from build123d import *

# Parameters (mm, degrees)
SKETCH1_R                = 0.15
BOSS_EXTRUDE1_DEPTH      = 0.1
SKETCH2_R                = 0.3
SKETCH2_R_2              = 0.15
BOSS_EXTRUDE2_DEPTH      = 0.1
BOSS_EXTRUDE2_DEPTH_BACK = 2
FILLET1_R                = 0.05
FILLET2_R                = 0.02
SKETCH3_R                = 0.431407551
SKETCH3_R_2              = 0.2
CUT_EXTRUDE1_DEPTH       = 1.9


with BuildPart() as part:
    # Sketch1 → Boss-Extrude1 (new body)
    with BuildSketch(Plane(origin=(0, 0, 0), x_dir=(1, 0, 0), z_dir=(0, 1, 0))):
        with BuildLine():
            Line((-82.406253285, -49.725868429), (-72.592962822, -38.875374501))
            ThreePointArc((-72.592962822, -38.875374501), (-71.888648973, -38.644732606), (-71.760288486, -37.914816674))
            Line((-71.760288486, -37.914816674), (-69.191054527, -35.004040233))
            Line((-69.191054527, -35.004040233), (-69.671325788, -34.569459042))
            Line((-69.671325788, -34.569459042), (-72.275341711, -37.469639173))
            ThreePointArc((-72.275341711, -37.469639173), (-72.996004438, -37.722822834), (-73.084190733, -38.481558565))
            Line((-73.084190733, -38.481558565), (-82.643859616, -49.510974991))
            Line((-82.643859616, -49.510974991), (-82.406253285, -49.725868429))
        make_face()
        with Locations((-72.433134731, -38.172736745)):
            Circle(SKETCH1_R, mode=Mode.SUBTRACT)
    extrude(amount=BOSS_EXTRUDE1_DEPTH)

    # Sketch2 → Boss-Extrude2 (add, two sides)
    with BuildSketch(Plane(origin=(0, 0.1, 0), x_dir=(1, 0, 0), z_dir=(0, 1, 0))) as boss_extrude2_sk:
        with Locations((-72.433134731, -38.172736745)):
            Circle(SKETCH2_R)
        with Locations((-72.433134731, -38.172736745)):
            Circle(SKETCH2_R_2, mode=Mode.SUBTRACT)
    extrude(amount=BOSS_EXTRUDE2_DEPTH)
    extrude(boss_extrude2_sk.sketch, amount=-BOSS_EXTRUDE2_DEPTH_BACK)

    # Fillet1
    fillet1_edges = [part.edges().sort_by_distance(p)[0] for p in [
        (-72.583134731, 0.2, 38.172736745),
        (-72.733134731, 0.2, 38.172736745),
    ]]
    fillet(fillet1_edges, radius=FILLET1_R)

    # Fillet2
    fillet2_edges = [part.edges().sort_by_distance(p)[0] for p in [
        (-77.499608053, 0.1, 44.300621465),
        (-71.888648973, 0.1, 38.644732606),
        (-70.475671506, 0.1, 36.459428453),
        (-69.431190157, 0.1, 34.786749638),
        (-70.973333749, 0.1, 36.019549108),
        (-72.733134731, 0.1, 38.172736745),
        (-72.996004438, 0.1, 37.722822834),
        (-77.864025175, 0.1, 43.996266778),
        (-82.52505645, 0.1, 49.61842171),
    ]]
    fillet(fillet2_edges, radius=FILLET2_R)

    # Sketch3 → Cut-Extrude1 (cut)
    with BuildSketch(Plane.XZ.offset(1.9)):
        with Locations((-72.433134731, 38.172736745)):
            Circle(SKETCH3_R)
        with Locations((-72.433134731, 38.172736745)):
            Circle(SKETCH3_R_2, mode=Mode.SUBTRACT)
    extrude(amount=-CUT_EXTRUDE1_DEPTH, mode=Mode.SUBTRACT)


solid = part.part
The listing builds one solid part. Answer for the finished solid, in the listing's coordinates (mm). Give positions to 0.01 mm unless a question says otherwise; leave off trailing zeros. Write each loop counter-clockwise with the first axis right and the second up, starting at its lowest first coordinate (ties: lowest second). Pieces come first, ordered by that corner, then holes. Notation, with made-up numbers: (53.5, 45.25) - (95.5, 45.25) arc R35 cw to (95.5, 79.25) - close; hole circle Ø1 at (21.25, 37). An arc over 180 degrees is marked (long way). Use a Markdown table: item, result.
1. Find the intervals of material crossed by probe 1 along X at (y, z) = (0.05, 45.25), in increasing order. Write a range as from..to.
Values follow:
| item | result |
|---|---|
| probe 1 | x = -78.95..-78.36 |
2. Section A-A on y = -0.9 is taken. Write down the section's boundary in (x, z).
Values follow:
| item | result |
|---|---|
| outline | circle Ø0.4 at (-72.43, 38.17); hole circle Ø0.3 at (-72.43, 38.17) |
3. Each of these flat-tipped pins is pushed along its axis until it touches: P1, Ø6.5, axis at x = -73.5, z = 42.5, coming from the -Y side; P2, Ø4, axis at x = -73, z = 40.5, coming from the +Y side; P3, Ø1, axis at x = -75.5, y = 0, coming from the -Z side. Where does it stop, or does it pass through?
Values follow:
| item | result |
|---|---|
| P1 | stops at y = 0 |
| P2 | stops at y = 0.1 |
| P3 | stops at z = 40.69 |
